from build123d import *

# Parameters (mm, degrees)
SKETCH1_W           = 50.8
SKETCH1_H           = 25.4
SKETCH1_W_2         = 44.45
SKETCH1_H_2         = 19.05
BOSS_EXTRUDE1_DEPTH = 1066.8
SKETCH2_R           = 14.2875
CUT_EXTRUDE1_DEPTH  = 1068.404590584
SKETCH3_R           = 3.175
CUT_EXTRUDE2_DEPTH  = 1068.404590584
SKETCH4_R           = 2.4638
CUT_EXTRUDE3_DEPTH  = 1068.404590584
SKETCH5_R           = 3.3734375
CUT_EXTRUDE4_DEPTH  = 1068.404590584
SKETCH6_R           = 3.3734375
CUT_EXTRUDE5_DEPTH  = 1068.404590584


with BuildPart() as part:
    # Sketch1 → Boss-Extrude1 (new body)
    with BuildSketch(Plane(origin=(0, 0, 0), x_dir=(1, 0, 0), z_dir=(0, 1, 0))):
        Rectangle(SKETCH1_W, SKETCH1_H)
        Rectangle(SKETCH1_W_2, SKETCH1_H_2, mode=Mode.SUBTRACT)
    extrude(amount=BOSS_EXTRUDE1_DEPTH)

    # Sketch2 → Cut-Extrude1 (cut, through all)
    with BuildSketch(Plane.XY.offset(12.7)):
        with Locations((0, 1041.4)):
            Circle(SKETCH2_R)
    extrude(amount=-CUT_EXTRUDE1_DEPTH, mode=Mode.SUBTRACT)

    # Sketch3 → Cut-Extrude2 (cut, through all)
    with BuildSketch(Plane.XY.offset(12.7)):
        with Locations((0, 12.7)):
            Circle(SKETCH3_R)
        with Locations((0, 38.1)):
            Circle(SKETCH3_R)
    extrude(amount=-CUT_EXTRUDE2_DEPTH, mode=Mode.SUBTRACT)

    # Sketch4 → Cut-Extrude3 (cut, through all)
    with BuildSketch(Plane.XY.offset(12.7)):
        with Locations((0, 977.9)):
            Circle(SKETCH4_R)
        with Locations((0, 952.5)):
            Circle(SKETCH4_R)
        with Locations((0, 927.1)):
            Circle(SKETCH4_R)
        with Locations((1.27, 519.585439926)):
            Circle(SKETCH4_R)
        with Locations((1.27, 494.185439926)):
            Circle(SKETCH4_R)
    extrude(amount=-CUT_EXTRUDE3_DEPTH, mode=Mode.SUBTRACT)

    # Sketch5 → Cut-Extrude4 (cut, through all)
    with BuildSketch(Plane.XY.offset(12.7)):
        with Locations((0, 76.2)):
            Circle(SKETCH5_R)
    extrude(amount=-CUT_EXTRUDE4_DEPTH, mode=Mode.SUBTRACT)

    # Sketch6 → Cut-Extrude5 (cut, through all)
    with BuildSketch(Plane.XY.offset(12.7)):
        with Locations((-17.78, 155.17537)):
            Circle(SKETCH6_R)
        with Locations((17.78, 155.17537)):
            Circle(SKETCH6_R)
    extrude(amount=-CUT_EXTRUDE5_DEPTH, mode=Mode.SUBTRACT)


solid = part.part
For this review, take the finished solid that the model builds, in its own axes (mm). A direction names the side the tool comes from. Coordinates: 2 decimals unless noted, no trailing zeros. Order: outer loops, then holes, each group sorted by start corner. A loop starts at its lowest first (then second) coordinate and runs counter-clockwise, first axis right, second up. Notation, with made-up numbers: (43, -32.75) -> (88, -32.75) arc R13 cw to (88, -14.75) -> close; hole circle Ø9 at (-18.75, 76). An arc over 180 degrees is marked (long way). Return JSON: item names as keys, results as strings.
1. The part is to be moulded in two halves that separate along Y. For faces 1 (the flat face through (0, 1066.8, -10)), 2 (the cylindrical face through (-1.86, 1055.566, 11.135)), 3 (the flat face through (22.225, 526, 0)), 4 (the cylindrical face through (-1.86, 1055.566, -11.09)), say which applies: +Y half, -Y half, draft (parallel to the pull), parting line (faces both ways), or undercut.
Answer block:
{"face 1": "+Y half", "face 2": "undercut", "face 3": "draft", "face 4": "undercut"}
2. For line 1 (Y direction, x = -17.78, z = -10.9); line 2 (X direction, y = 1024, z = 8.75) (3 decimals); line 3 (Z direction, x = 15.5, y = 288) (3 decimals), list the stretches that pass through material, from the lowest coordinate up. Write a range as from..to.
Answer block:
{"line 1": "0..151.8, 158.55..1066.8", "line 2": "-25.4..-22.225, 22.225..25.4", "line 3": "-12.7..-9.525, 9.525..12.7"}
3. We need section C-C on y = 398.5. Write out the cut boundary in (x, z) (3 decimals), and give its area (3 significant figures).
Answer block:
{"outline": "(-25.4, -12.7) -> (25.4, -12.7) -> (25.4, 12.7) -> (-25.4, 12.7) -> close; hole (-22.225, -9.525) -> (22.225, -9.525) -> (22.225, 9.525) -> (-22.225, 9.525) -> close", "area": "444 mm²"}
4. We need section B-B on z = 1.5. Write out the cut boundary in (x, y) (3 decimals), and give its area (3 significant figures).
Answer block:
{"outline": "(-25.4, 0) -> (-22.225, 0) -> (-22.225, 1066.8) -> (-25.4, 1066.8) -> close; (22.225, 0) -> (25.4, 0) -> (25.4, 1066.8) -> (22.225, 1066.8) -> close", "area": "6,770 mm²"}
5. We need section A-A on y = 1041.4. Write out the cut boundary in (x, z) (1 decimal).
Answer block:
{"outline": "(-25.4, -12.7) -> (-14.3, -12.7) -> (-14.3, -9.5) -> (-22.2, -9.5) -> (-22.2, 9.5) -> (-14.3, 9.5) -> (-14.3, 12.7) -> (-25.4, 12.7) -> close; (14.3, -12.7) -> (25.4, -12.7) -> (25.4, 12.7) -> (14.3, 12.7) -> (14.3, 9.5) -> (22.2, 9.5) -> (22.2, -9.5) -> (14.3, -9.5) -> close"}
6. Machinability: for faces 5 (the flat face through (-22.225, 526, 0)), 6 (the flat face through (0, 526, -12.7)), which of the approach directions +Z, -Z, +X, -X, +Y, -Y give a long, thin tool a straight path to every point of the face, cutting with its end or side? Answer none if there is none.
Answer block:
{"face 5": "+Y, -Y", "face 6": "-Z, +X, -X, +Y, -Y"}
